Source: CAD feature listing. Evaluate the final solid. Frame: model axes, mm. A direction names the side the tool comes from. Give positions to 0.01 mm unless a question says otherwise; leave off trailing zeros. Loops run counter-clockwise (first coordinate to the right, second up) from the corner with the lowest first, then second, coordinate; pieces in that order, holes last. Notation, with made-up numbers: M 10,67.25 L 20,67.25 A37 ccw 20,106.25 Z; hole C -21.5,84 d10. An arc over 180 degrees is marked long. Answer in a Markdown table with one row per item.
```python
from build123d import *

# Parameters (mm, degrees)
CROQUIS1_R              = 29
CROQUIS1_R_2            = 2.75
CROQUIS1_R_3            = 12
SALIENTE_EXTRUIR1_DEPTH = 8
CROQUIS2_R              = 16
CROQUIS2_R_2            = 12
SALIENTE_EXTRUIR2_DEPTH = 4
SALIENTE_EXTRUIR3_START = -4
CROQUIS3_R              = 12
CROQUIS3_R_2            = 11
SALIENTE_EXTRUIR3_DEPTH = 4
REDONDEO2_R             = 0.5


with BuildPart() as part:
    # Croquis1 → Saliente-Extruir1 (new body)
    with BuildSketch(Plane.XY):
        Circle(CROQUIS1_R)
        with Locations((-15.5, 15.5)):
            Circle(CROQUIS1_R_2, mode=Mode.SUBTRACT)
        with Locations((15.5, 15.5)):
            Circle(CROQUIS1_R_2, mode=Mode.SUBTRACT)
        with Locations((15.5, -15.5)):
            Circle(CROQUIS1_R_2, mode=Mode.SUBTRACT)
        with Locations((-15.5, -15.5)):
            Circle(CROQUIS1_R_2, mode=Mode.SUBTRACT)
        Circle(CROQUIS1_R_3, mode=Mode.SUBTRACT)
    extrude(amount=-SALIENTE_EXTRUIR1_DEPTH)

    # Croquis2 → Saliente-Extruir2 (add)
    with BuildSketch(Plane(origin=(0, 0, -8), x_dir=(-1, 0, 0), z_dir=(0, 0, -1))):
        with Locations(Location((0, 0, 0), (0, 0, 180))):
            Circle(CROQUIS2_R)
        with Locations(Location((0, 0, 0), (0, 0, 180))):
            Circle(CROQUIS2_R_2, mode=Mode.SUBTRACT)
    extrude(amount=SALIENTE_EXTRUIR2_DEPTH)

    # Croquis3 → Saliente-Extruir3 (add)
    with BuildSketch(Plane(origin=(0, 0, -4), x_dir=(-1, 0, 0), z_dir=(0, 0, -1)).offset(SALIENTE_EXTRUIR3_START)):
        Circle(CROQUIS3_R)
        Circle(CROQUIS3_R_2, mode=Mode.SUBTRACT)
    extrude(amount=SALIENTE_EXTRUIR3_DEPTH)

    # Redondeo2
    redondeo2_edges = [part.edges().sort_by_distance(p)[0] for p in [
        (-16, 0, -12),
        (-12, 0, -12),
        (-29, 0, -8),
    ]]
    fillet(redondeo2_edges, radius=REDONDEO2_R)


solid = part.part
```
Q1. Mould query, pull axis X, two halves, no side actions, for faces 1 (the flat face through (-12, 0, 0)), 2 (the cylindrical face through (-18.247, -15.379, -3.944)), 3 (the cylindrical face through (13.38, -25.73, -3.7)). Classes: +X half, -X half, draft (parallel to the pull), parting line (faces both ways), or undercut.
Values follow:
| item | result |
|---|---|
| face 1 | draft |
| face 2 | undercut |
| face 3 | parting line |
Q2. Section query A-A (x = 0). Output: boundary loops of the cut face in (y, z), plus the area to 3 significant figures.
Values follow:
| item | result |
|---|---|
| outline | M -29,-7.5 A0.5 ccw -28.5,-8 L -16,-8 L -16,-11.5 A0.5 ccw -15.5,-12 L -12.5,-12 A0.5 ccw -12,-11.5 L -12,-4 L -11,-4 L -11,0 L -29,0 Z; M 11,-4 L 12,-4 L 12,-11.5 A0.5 ccw 12.5,-12 L 15.5,-12 A0.5 ccw 16,-11.5 L 16,-8 L 28.5,-8 A0.5 ccw 29,-7.5 L 29,0 L 11,0 Z |
| area | 312 mm^2 |
Q3. Contact query for flat-ended pins moving along their axis: pin 1 Ø6 at (y, z) = (17, -9) entering from -X; pin 2 Ø4 at (x, z) = (2, -4.5) entering from +Y; pin 3 Ø4.5 at (x, y) = (15.5, 15.5) entering from -Z; pin 4 Ø4 at (y, z) = (4, -9) entering from -X. Output: stop coordinate, or through.
Values follow:
| item | result |
|---|---|
| pin 1 | x = -25.19 |
| pin 2 | y = 29 |
| pin 3 | through |
| pin 4 | x = -28.88 |
Q4. Section query D-D (z = -2.25). Output: boundary loops of the cut face in (x, y).
Values follow:
| item | result |
|---|---|
| outline | C 0,0 d58; hole C -15.5,-15.5 d5.5; hole C -15.5,15.5 d5.5; hole C 0,0 d22; hole C 15.5,-15.5 d5.5; hole C 15.5,15.5 d5.5 |
Q5. Section query B-B (z = -6). Output: boundary loops of the cut face in (x, y), plus the area to 3 significant figures.
Values follow:
| item | result |
|---|---|
| outline | C 0,0 d58; hole C -15.5,-15.5 d5.5; hole C -15.5,15.5 d5.5; hole C 0,0 d24; hole C 15.5,-15.5 d5.5; hole C 15.5,15.5 d5.5 |
| area | 2,090 mm^2 |
Q6. Ray query, probe 1 along Y at (x, z) = (0, -9.4); probe 2 along Y at (x, z) = (15.5, -4); probe 3 along Y at (x, z) = (0, -2.2). Return the intervals inside material, ascending. Write a range as from..to.
Values follow:
| item | result |
|---|---|
| probe 1 | -16..-12, 12..16 |
| probe 2 | -24.51..-18.25, -12.75..12.75, 18.25..24.51 |
| probe 3 | -29..-11, 11..29 |
Q7. Reachability of faces 4 (the flat face through (12, -12, -8)), 5 (the cylindrical face through (-15.858, 18.227, -3.944)) from +Z, -Z, +X, -X, +Y, -Y: full face, straight path, thin tool, end or side. Return the list, or none.
Values follow:
| item | result |
|---|---|
| face 4 | -Z |
| face 5 | +Z, -Z |
